Verification items for the finished model (mm, model axes). Round coordinates to 2 decimals unless told otherwise and drop trailing zeros. Order: outer loops, then holes, each group sorted by start corner. A loop starts at its lowest first (then second) coordinate and runs counter-clockwise, first axis right, second up. Notation, with made-up numbers: (46.25, -8.5) -> (72.25, -8.5) arc R12 cw to (72.25, 13.5) -> close; hole circle Ø2 at (-6, 52). An arc over 180 degrees is marked (long way). Put each result on its own line as item: value.
```python
from build123d import *

# Parameters (mm, degrees)
F0_R     = 25
F1_DEPTH = 880
F2_R     = 5
F3_DEPTH = 3
F4_R     = 5
F5_DEPTH = 3


with BuildPart() as f1:
    # F0 (on Front) → F1 (new body)
    with BuildSketch(Plane.XZ):
        Circle(F0_R)
    extrude(amount=F1_DEPTH)

    # F2 (on face) → F3 (join)
    with BuildSketch(Plane.XZ.offset(880)):
        with BuildLine():
            Line((10, 55), (-10, 55))
            Line((-10, 55), (-10, 22.912878))
            ThreePointArc((-10, 22.912878), (0, 25), (10, 22.912878))
            Line((10, 22.912878), (10, 55))
        make_face()
        with Locations((0.225252, 44.60642)):
            Circle(F2_R, mode=Mode.SUBTRACT)
        with BuildLine():
            ThreePointArc((10, 22.912878), (0, 25), (-10, 22.912878))
            Line((-10, 22.912878), (-10, -5))
            Line((-10, -5), (10, -5))
            Line((10, -5), (10, 22.912878))
        make_face()
    extrude(amount=F3_DEPTH)

    # F4 (on face) → F5 (join)
    with BuildSketch(Plane(origin=(0, 0, 0), x_dir=(-1, 0, 0), z_dir=(0, 1, 0))):
        with BuildLine():
            ThreePointArc((10, 22.912878), (0, 25), (-10, 22.912878))
            Line((-10, 22.912878), (-10, -5))
            Line((-10, -5), (10, -5))
            Line((10, -5), (10, 22.912878))
        make_face()
        with BuildLine():
            Line((10, 55), (-10, 55))
            Line((-10, 55), (-10, 22.912878))
            ThreePointArc((-10, 22.912878), (0, 25), (10, 22.912878))
            Line((10, 22.912878), (10, 55))
        make_face()
        with Locations((-0.179578, 44.637514)):
            Circle(F4_R, mode=Mode.SUBTRACT)
    extrude(amount=F5_DEPTH)


solid = f1.part
```
Item 1: Depth check by flat-ended pin: pin 1 Ø12 at (y, z) = (-190.5, -0.5) entering from +X; pin 2 Ø2.5 at (y, z) = (1, 40) entering from -X; pin 3 Ø0.9 at (x, y) = (0.5, -881.5) entering from -Z; pin 4 Ø12 at (x, z) = (-9, -16.5) entering from -Y. Enter the tip coordinate at first touch or a pass-through.
Geometry check:
pin 1: x = 25
pin 2: x = -10
pin 3: z = -5
pin 4: y = -880
Item 2: Material ranges on line 1 along Y through (x, z) = (8.5, 33.5); line 2 along Z through (x, y) = (1.5, -53); line 3 along Y through (x, z) = (-14.5, 8), recorded low to high.
Geometry check:
line 1: -883 to -880, 0 to 3
line 2: -24.95 to 24.95
line 3: -880 to 0
Item 3: Sectioned sample at A-A, the plane y = -550. Record the boundary of the cut face in (x, z).
Geometry check:
outline: circle Ø50 at (0, 0)
